CAD build for the part. Positions are in the model's coordinates, mm. Give positions to 0.01 mm unless a question says otherwise; leave off trailing zeros. Loops run counter-clockwise (first coordinate to the right, second up) from the corner with the lowest first, then second, coordinate; pieces in that order, holes last. Notation, with made-up numbers: (70, 22.5) - (82, 22.5) arc R7 ccw to (82, 33.5) - close; hole circle Ø11 at (54.25, 43). An arc over 180 degrees is marked (long way). Return JSON: item names as keys, results as strings.
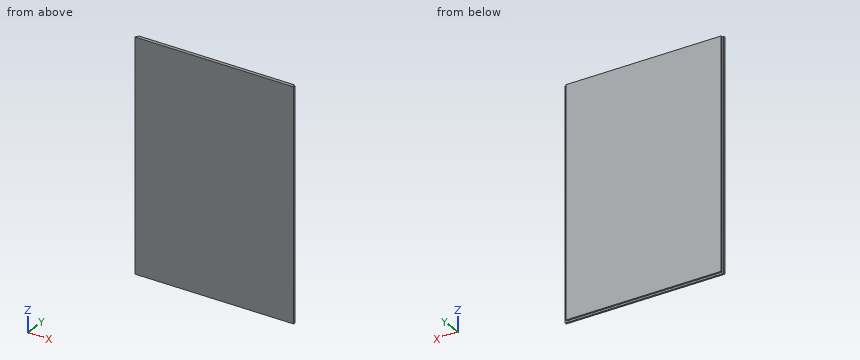
from build123d import *

# Parameters (mm, degrees)
SKETCH1_W               = 298.45
SKETCH1_H               = 431.165
BOSS_EXTRUDE1_DEPTH     = 6.35
CUT_EXTRUDE1_DEPTH      = 525.419662317
CUT_EXTRUDE1_DEPTH_BACK = 3.175


with BuildPart() as part:
    # Sketch1 → Boss-Extrude1 (new body)
    with BuildSketch(Plane(origin=(0, 0, 0), x_dir=(1, 0, 0), z_dir=(0, 1, 0))):
        with Locations((149.225, 215.5825)):
            Rectangle(SKETCH1_W, SKETCH1_H)
    extrude(amount=BOSS_EXTRUDE1_DEPTH)

    # Sketch2 → Cut-Extrude1 (cut, two sides: drawn at the far end of the back side and taken through both)
    with BuildSketch(Plane(origin=(0, 6.35, 0), x_dir=(1, 0, 0), z_dir=(0, 1, 0)).offset(-CUT_EXTRUDE1_DEPTH_BACK)):
        Polygon((0, 0), (3.175, 0), (3.175, 427.99), (295.275, 427.99), (295.275, 0), (298.45, 0), (298.45, 431.165), (0, 431.165), align=None)
    extrude(amount=CUT_EXTRUDE1_DEPTH + CUT_EXTRUDE1_DEPTH_BACK, mode=Mode.SUBTRACT)


solid = part.part
1. Drill centre lines: probe 1 along X at (y, z) = (5.75, -271) (3 decimals); probe 2 along Z at (x, y) = (269, 6.25). Where is each one in solid material? Low to high.
Values follow:
{"probe 1": "x = 3.175 to 295.275", "probe 2": "z = -427.99 to 0"}
2. Drop flat-ended pins along their axis: P1, Ø1, axis at y = 4.5, z = -115.5, coming from the -X side (3 decimals); P2, Ø3, axis at x = 60, y = 5.5, coming from the -Z side; P3, Ø3.5, axis at y = 5, z = -211.5, coming from the +X side (3 decimals). Give the stop position or say it passes through.
Values follow:
{"P1": "stops at x = 3.175", "P2": "stops at z = -427.99", "P3": "stops at x = 295.275"}
3. Cut at A-A, the plane y = 5.25. Write the cut outline in (x, z) (3 decimals).
Values follow:
{"outline": "(3.175, -427.99) - (295.275, -427.99) - (295.275, 0) - (3.175, 0) - close"}
